CAD build for the part. Positions are in the model's coordinates, mm. Face numbers are marked on the shaded views. A direction names the side the tool comes from. Coordinates: 2 decimals unless noted, no trailing zeros. Order: outer loops, then holes, each group sorted by start corner. A loop starts at its lowest first (then second) coordinate and runs counter-clockwise, first axis right, second up. Notation, with made-up numbers: (40.25, 36) - (47.25, 36) arc R28 cw to (47.25, 54) - close; hole circle Ø8 at (-37, -14.5). An arc over 180 degrees is marked (long way). Return JSON: item names as keys, results as strings.
from build123d import *

# Parameters (mm, degrees)
F_9_64_ALLEN_DEPTH = 3.175


with BuildPart() as part:
    # Sketch1 → Revolve1 (revolve)
    with BuildSketch(Plane(origin=(0, 0, 0), x_dir=(1, 0, 0), z_dir=(0, 1, 0))):
        Polygon((0, 0), (0, 26.3906), (2.0828, 26.3906), (2.0828, 4.1656), (3.429, 4.1656), (3.429, 0), align=None)
    revolve(axis=Axis((0, 0, 0), (0, 0, -1)))

    # Sketch2 → 9-64 allen (cut)
    with BuildSketch(Plane.XY):
        Polygon((2.062222993, 0), (1.031111496, 1.7859375), (-1.031111496, 1.7859375), (-2.062222993, 0), (-1.031111496, -1.7859375), (1.031111496, -1.7859375), align=None)
    extrude(amount=-F_9_64_ALLEN_DEPTH, mode=Mode.SUBTRACT)


solid = part.part
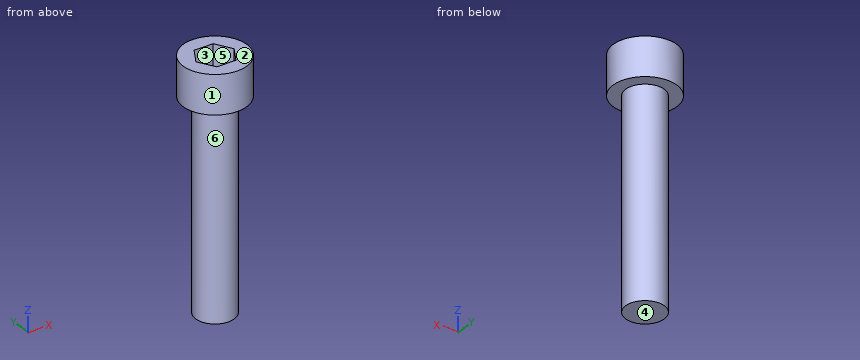
Item 1: Band-saw the part on C-C, the plane y = -0.75. List the corners of the cut face in (x, z) (3 decimals), then the cut area to 3 significant figures.
Findings below:
{"outline": "(-3.346, -4.166) - (-1.943, -4.166) - (-1.943, -26.391) - (1.943, -26.391) - (1.943, -4.166) - (3.346, -4.166) - (3.346, 0) - (1.629, 0) - (1.629, -3.175) - (-1.629, -3.175) - (-1.629, 0) - (-3.346, 0) - close", "area": "104 mm²"}
Item 2: Band-saw the part on D-D, the plane z = -17. List the corners of the cut face in (x, y).
Findings below:
{"outline": "circle Ø4.17 at (0, 0)"}
Item 3: Wall check: L1, parallel to Z at x = 2.25, y = 0.5; L2, parallel to Z at x = -0.5, y = 0.25 (3 decimals); L3, parallel to Y at x = 0, z = -11. Give the ranges that are in metal, low to high. Write a range as [from, to].
Findings below:
{"L1": "z = [-4.17, 0]", "L2": "z = [-26.391, -3.175]", "L3": "y = [-2.08, 2.08]"}
Item 4: Band-saw the part on A-A, the plane z = -2.5. List the corners of the cut face in (x, y), then the cut area to 3 significant figures.
Findings below:
{"outline": "circle Ø6.86 at (0, 0); hole (-2.06, 0) - (-1.03, -1.79) - (1.03, -1.79) - (2.06, 0) - (1.03, 1.79) - (-1.03, 1.79) - close", "area": "25.9 mm²"}
Item 5: Which spindle directions (+Z, -Z, +X, -X, +Y, -Y) get a long thin tool onto all of the face, cutting with end or side? Do the marked faces 4, 5 and 6. Say none if no direction does.
Findings below:
{"face 4": "-Z, +X, -X, +Y, -Y", "face 5": "+Z", "face 6": "-Z"}
Item 6: Band-saw the part on B-B, the plane x = 0. List the corners of the cut face in (y, z) (3 decimals).
Findings below:
{"outline": "(-3.429, -4.166) - (-2.083, -4.166) - (-2.083, -26.391) - (2.083, -26.391) - (2.083, -4.166) - (3.429, -4.166) - (3.429, 0) - (1.786, 0) - (1.786, -3.175) - (-1.786, -3.175) - (-1.786, 0) - (-3.429, 0) - close"}
Item 7: Drop flat-ended pins along their axis: P1, Ø1.1, axis at x = -0.5, y = 0, coming from the +Z side (3 decimals); P2, Ø4, axis at y = 2.5, z = -9.5, coming from the -X side; P3, Ø0.6, axis at x = -0.5, z = -1, coming from the -Y side. Give the stop position or say it passes through.
Findings below:
{"P1": "stops at z = -3.175", "P2": "stops at x = -2.02", "P3": "stops at y = -3.42"}
Item 8: Mould opens along Y. For the marked faces 1, 2 and 3 say: released by +Y, released by -Y, zero draft, split by the parting line, or undercut.
Findings below:
{"face 1": "split by the parting line", "face 2": "zero draft", "face 3": "undercut"}
